Design review of the part built by this model. Coordinates are the model's own, in mm. Face numbers are marked on the shaded views. A direction names the side the tool comes from. Round coordinates to 2 decimals unless told otherwise and drop trailing zeros. Order: outer loops, then holes, each group sorted by start corner. A loop starts at its lowest first (then second) coordinate and runs counter-clockwise, first axis right, second up. Notation, with made-up numbers: M 29.25,50.25 L 60.25,50.25 A33 ccw 60.25,79.25 Z; hole C 83,77.25 d1. An arc over 180 degrees is marked long. Use a Markdown table: item, result. Add a question column.
(1) Take a section at B-B (z = 0). Write out the cut boundary in (x, y), then the cut area to 3 significant figures.
(2) For pin 1 (3 mm diameter, centred on x = 54, y = 43, fed in from +Z); pin 2 (10 mm diameter, centred on y = 11, z = -11.5, fed in from +X); pin 3 (21 mm diameter, centred on x = 82.5, y = 52, fed in from +Z); pin 4 (10 mm diameter, centred on y = 37.5, z = -20.5, fed in from -X), all flat-tipped, find the tip position at first contact; note any pin that passes through.
(3) Machinability: for the marked faces 1, 2, 3 and 4, which of the approach directions +Z, -Z, +X, -X, +Y, -Y give a long, thin tool a straight path to every point of the face, cutting with its end or side? Answer none if there is none.
(4) Take a section at C-C (y = 40.5). Write out the cut boundary in (x, z).
(5) The part is to be moulded in two halves that separate along Y. For the marked faces 5, 6 and 7, say which applies: released by +Y, released by -Y, zero draft, split by the parting line, or undercut.
(6) Take a section at D-D (y = 25). Write out the cut boundary in (x, z), then the cut area to 3 significant figures.
(7) Take a section at A-A (x = -20). Write out the cut boundary in (y, z).
(8) To check wall thickness, follow probe 1 along Z at (x, y) = (-20, 65); probe 2 along Y at (x, z) = (-14, 19); probe 3 along Z at (x, y) = (48, 54.5). State the ranges of each line that lie inside material, in increasing order. Write a range as from..to.
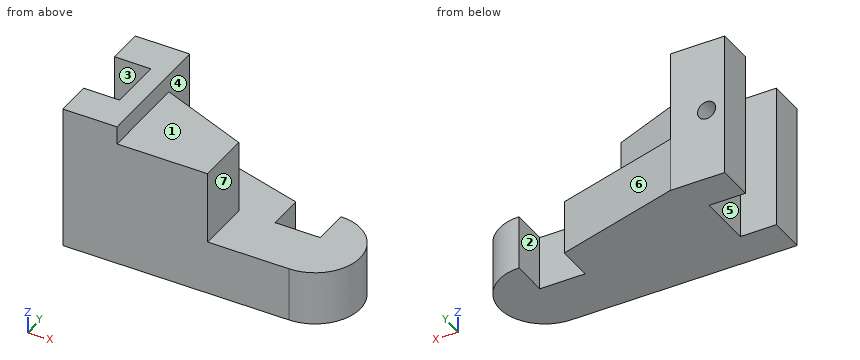
```python
from build123d import *

# Parameters (mm, degrees)
BOSS_EXTRUDE1_DEPTH        = 40
BOSS_EXTRUDE2_START        = -40
BOSS_EXTRUDE2_DEPTH        = 30
BOSS_EXTRUDE3_DEPTH        = 40
F_10_0MM_DOWEL_HOLE1_D     = 10
F_10_0MM_DOWEL_HOLE1_DEPTH = 20


with BuildPart() as part:
    # Sketch1 → Boss-Extrude1 (new, symmetric)
    with BuildSketch(Plane.XY):
        Polygon((0, 0), (0, 70), (-30, 70), (-30, 50), (-10, 50), (-10, 20), (-30, 20), (-30, 0), align=None)
    extrude(amount=BOSS_EXTRUDE1_DEPTH, both=True)

    # Sketch1<3> → Boss-Extrude2 (add)
    with BuildSketch(Plane.XY.offset(BOSS_EXTRUDE2_START)):
        Polygon((0, 70), (-30, 70), (-30, 50), (-10, 50), (-10, 20), (-30, 20), (-30, 0), (0, 0), align=None)
        with BuildLine():
            Line((70, 50), (0, 70))
            Line((0, 70), (0, 0))
            Line((0, 0), (95, 0))
            ThreePointArc((95, 0), (120, 25), (95, 50))
            Line((95, 50), (95, 30))
            Line((95, 30), (70, 30))
            Line((70, 30), (70, 50))
        make_face()
    extrude(amount=BOSS_EXTRUDE2_DEPTH)

    # Sketch2 → Boss-Extrude3 (add)
    with BuildSketch(Plane.XY.offset(-10)):
        Polygon((0, 50), (0, 0), (50, 0), (50, 30), align=None)
    extrude(amount=BOSS_EXTRUDE3_DEPTH)

    # Ø10.0mm Dowel Hole1
    with Locations(Plane(origin=(0, 70, 0), x_dir=(1, 0, 0), z_dir=(0, 1, 0))):
        with Locations((-20, 0)):
            Hole(F_10_0MM_DOWEL_HOLE1_D / 2, depth=F_10_0MM_DOWEL_HOLE1_DEPTH)


solid = part.part
```
Verdict:
| question | item | result |
|---|---|---|
| 1 | outline | M -30,0 L 50,0 L 50,30 L 0,50 L 0,70 L -15,70 L -15,50 L -10,50 L -10,20 L -30,20 Z; M -30,50 L -25,50 L -25,70 L -30,70 Z |
| 1 | area | 3,300 mm^2 |
| 2 | pin 1 | stops at z = -10 |
| 2 | pin 2 | stops at x = 118.32 |
| 2 | pin 3 | passes through |
| 2 | pin 4 | stops at x = -10 |
| 3 | face 1 | +Z, +X, +Y, -Y |
| 3 | face 2 | +Z, -Z, +Y |
| 3 | face 3 | +Z, -Z, -X |
| 3 | face 4 | +Z, +X, +Y |
| 4 | outline | M -10,-40 L 70,-40 L 70,-10 L 23.75,-10 L 23.75,30 L 0,30 L 0,40 L -10,40 Z; M 95,-40 L 114.62,-40 L 114.62,-10 L 95,-10 Z |
| 5 | face 5 | undercut |
| 5 | face 6 | released by +Y |
| 5 | face 7 | zero draft |
| 6 | outline | M -10,-40 L 120,-40 L 120,-10 L 50,-10 L 50,30 L 0,30 L 0,40 L -10,40 Z |
| 6 | area | 6,400 mm^2 |
| 7 | outline | M 0,-40 L 20,-40 L 20,40 L 0,40 Z; M 50,-40 L 70,-40 L 70,-5 L 50,-5 Z; M 50,5 L 70,5 L 70,40 L 50,40 Z |
| 8 | probe 1 | z = -40..-5, 5..40 |
| 8 | probe 2 | y = 0..20, 50..70 |
| 8 | probe 3 | z = -40..-10 |
